```python
from build123d import *

# Parameters (mm, degrees)
EXTRUDE_1_DEPTH     = 60
CUT_EXTRUDE_1_DEPTH = 66
CUT_EXTRUDE_2_DEPTH = 5
CUT_EXTRUDE_START   = -5
CUT_EXTRUDE_3_DEPTH = 5
SKETCH_6_W          = 20
SKETCH_6_H          = 20
CUT_EXTRUDE_4_DEPTH = 5
CUT_EXTRUDE_5_DEPTH = 30


with BuildPart() as part:
    # 草图1 → 凸台-拉伸1 (new body)
    with BuildSketch(Plane(origin=(0, 0, 0), x_dir=(1, 0, 0), z_dir=(0, 1, 0))):
        Polygon((10, 4.142135624), (4.142135624, 10), (-4.142135624, 10), (-10, 4.142135624), (-10, -4.142135624), (-4.142135624, -10), (4.142135624, -10), (10, -4.142135624), align=None)
    extrude(amount=EXTRUDE_1_DEPTH)

    # 草图2 → 切除-拉伸1 (cut)
    with BuildSketch(Plane.XY.offset(10)):
        with BuildLine():
            Line((-10, 10), (-10, -2.389295552))
            Line((-10, -2.389295552), (10, -2.389295552))
            Line((10, -2.389295552), (10, 10))
            ThreePointArc((10, 10), (0, 0), (-10, 10))
        make_face()
    extrude(amount=-CUT_EXTRUDE_1_DEPTH, mode=Mode.SUBTRACT)

    # 草图4 → 切除-拉伸2 (cut)
    with BuildSketch(Plane.XY.offset(10)):
        with BuildLine():
            Line((-10, 10), (-10, 20))
            Line((-10, 20), (10, 20))
            Line((10, 20), (10, 10))
            ThreePointArc((10, 10), (0, 0), (-10, 10))
        make_face()
    extrude(amount=-CUT_EXTRUDE_2_DEPTH, mode=Mode.SUBTRACT)

    # 草图5 → 切除-拉伸3 (cut)
    with BuildSketch(Plane(origin=(0, 0, -10), x_dir=(-1, 0, 0), z_dir=(0, 0, -1)).offset(CUT_EXTRUDE_START)):
        with BuildLine():
            Line((-10, 10), (-10, 20))
            Line((-10, 20), (10, 20))
            Line((10, 20), (10, 10))
            ThreePointArc((10, 10), (0, 0), (-10, 10))
        make_face()
    extrude(amount=CUT_EXTRUDE_3_DEPTH, mode=Mode.SUBTRACT)

    # 草图6 → 切除-拉伸4 (cut, symmetric)
    with BuildSketch(Plane.XY):
        with Locations((0, 50)):
            Rectangle(SKETCH_6_W, SKETCH_6_H)
    extrude(amount=CUT_EXTRUDE_4_DEPTH, both=True, mode=Mode.SUBTRACT)

    # 草图7 → 切除-拉伸5 (cut)
    with BuildSketch(Plane.XY.offset(10)):
        with BuildLine():
            Line((-10, 50), (-10, 63.661192365))
            Line((-10, 63.661192365), (10, 63.661192365))
            Line((10, 63.661192365), (10, 50))
            ThreePointArc((10, 50), (0, 60), (-10, 50))
        make_face()
    extrude(amount=-CUT_EXTRUDE_5_DEPTH, mode=Mode.SUBTRACT)


solid = part.part
```
Geometry: final body of the model. Coordinates: model frame, mm. A direction names the side the tool comes from. Round coordinates to 2 decimals unless told otherwise and drop trailing zeros. Loops run counter-clockwise (first coordinate to the right, second up) from the corner with the lowest first, then second, coordinate; pieces in that order, holes last. Notation, with made-up numbers: (44, 7) -> (50, 7) arc R26 cw to (50, 26) -> close; hole circle Ø3 at (1.5, -3). An arc over 180 degrees is marked (long way). Use one line per item in the form item = value. Start each with the question number.
1) Line query: L1, parallel to Z at x = -0.5, y = 44; L2, parallel to Y at x = 0, z = 8; L3, parallel to Z at x = 5.5, y = 47. Output: solid intervals per line, ascending.
2) Draft query along Z for faces 5 (the flat face through (0, 50, -5)), 6 (the flat face through (-7.11, 38.06, 7.03)), 7 (the flat face through (0, 20, 7)), 8 (the flat face through (7.11, 38.06, -7.03)). Return one class per face: released by +Z, released by -Z, zero draft, split by the parting line, or undercut.
3) Section B-B on x = 0. Output: boundary loops of the cut face in (y, z), then the cut area to 3 significant figures.
4) Section C-C on x = 5.5. Output: boundary loops of the cut face in (y, z), then the cut area to 3 significant figures.
5) Access query for faces 1 (the flat face through (0, 50, 5)), 2 (the flat face through (0, 10, 5)), 3 (the flat face through (0, 40, 10)), 4 (the flat face through (0, 20, -7)). Directions: +Z, -Z, +X, -X, +Y, -Y. A direction counts if a zero-diameter tool reaches every point of the face in a straight line with its end or side. Return the directions, or none.
6) First-contact query: P1, Ø3, axis at y = 52, z = -5, coming from the -X side; P2, Ø5, axis at x = 4.5, z = 1.5, coming from the +Y side; P3, Ø2, axis at x = -4, y = 12.5, coming from the +Z side. Flat tips, straight axial feed; report the tip coordinate or a pass-through.
7) Section A-A on y = 23.5. Output: boundary loops of the cut face in (x, z), then the cut area to 3 significant figures.
8) Section D-D on z = 7. Output: boundary loops of the cut face in (x, y).
Response:
q1.L1 = -10 to -5, 5 to 10
q1.L2 = 20 to 60
q1.L3 = -8.64 to -5, 5 to 8.64
q2.face_5 = undercut
q2.face_6 = released by +Z
q2.face_7 = zero draft
q2.face_8 = released by -Z
q3.outline = (0, -5) -> (20, -5) -> (20, -10) -> (60, -10) -> (60, -5) -> (40, -5) -> (40, 5) -> (60, 5) -> (60, 10) -> (20, 10) -> (20, 5) -> (0, 5) -> close
q3.area = 800 mm^2
q4.outline = (1.65, -5) -> (20, -5) -> (20, -8.64) -> (58.35, -8.64) -> (58.35, -5) -> (40, -5) -> (40, 5) -> (58.35, 5) -> (58.35, 8.64) -> (20, 8.64) -> (20, 5) -> (1.65, 5) -> close
q4.area = 663 mm^2
q5.face_1 = +X, -X, +Y
q5.face_2 = +Z, +X, -X, -Y
q5.face_3 = +Z, +X, -X, +Y, -Y
q5.face_4 = -Z, +X, -X, -Y
q6.P1 = -9.14
q6.P2 = 40
q6.P3 = 5
q7.outline = (-10, -4.14) -> (-4.14, -10) -> (4.14, -10) -> (10, -4.14) -> (10, 4.14) -> (4.14, 10) -> (-4.14, 10) -> (-10, 4.14) -> close
q7.area = 331 mm^2
q8.outline = (-7.14, 20) -> (7.14, 20) -> (7.14, 57) arc R10 ccw to (-7.14, 57) -> close
